Source: three-view drawing plus pictorial views. Frame: mm from the lowest corner of the part. Give positions to 0.01 mm unless a question says otherwise; leave off trailing zeros. Loops run counter-clockwise (first coordinate to the right, second up) from the corner with the lowest first, then second, coordinate; pieces in that order, holes last. Notation, with made-up numbers: (49.5, -28) - (92.5, -28) arc R19 ccw to (92.5, -5) - close; hole circle Ø8 at (9, 82). An arc over 180 degrees is marked (long way). Put each result on its own line as item: value.
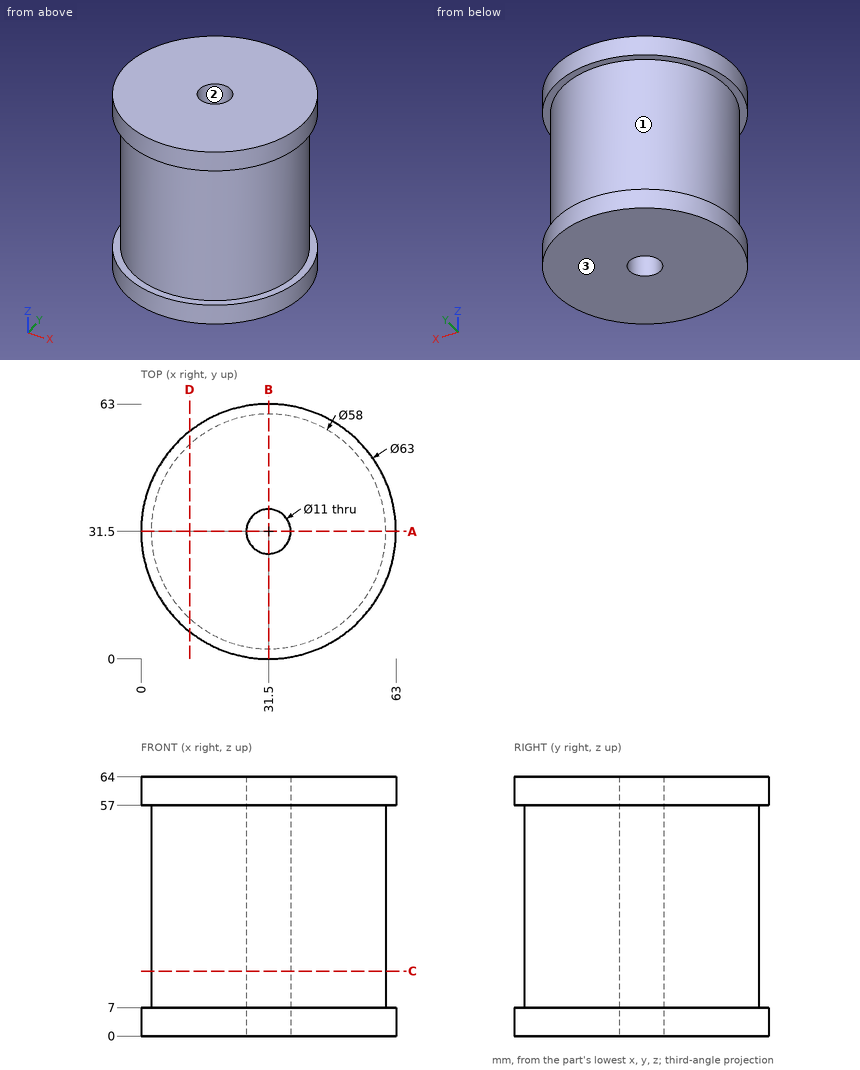
1) Pin query (flat end, axial travel): P1, Ø10, axis at x = 17.5, z = 10, coming from the -Y side; P2, Ø2, axis at y = 7.5, z = 27.5, coming from the +X side; P3, Ø1, axis at y = 25.5, z = 22, coming from the +X side; P4, Ø6.5, axis at x = 31.5, y = 31.5, coming from the -Z side. Return the tip coordinate at first contact, or that it passes through.
Check result:
P1: y = 1.63
P2: x = 49.16
P3: x = 59.97
P4: through
2) Section query A-A, the plane y = 31.5. Output: boundary loops of the cut face in (x, z).
Check result:
outline: (0, 0) - (26, 0) - (26, 64) - (0, 64) - (0, 57) - (2.5, 57) - (2.5, 7) - (0, 7) - close; (37, 0) - (63, 0) - (63, 7) - (60.5, 7) - (60.5, 57) - (63, 57) - (63, 64) - (37, 64) - close
3) Section query D-D, the plane x = 12. Output: boundary loops of the cut face in (y, z), plus the area to 3 significant figures.
Check result:
outline: (6.76, 0) - (56.24, 0) - (56.24, 7) - (52.97, 7) - (52.97, 57) - (56.24, 57) - (56.24, 64) - (6.76, 64) - (6.76, 57) - (10.03, 57) - (10.03, 7) - (6.76, 7) - close
area: 2,840 mm²
4) Section query C-C, the plane z = 16. Output: boundary loops of the cut face in (x, y).
Check result:
outline: circle Ø58 at (31.5, 31.5); hole circle Ø11 at (31.5, 31.5)
5) Material intervals for line 1 along Y through (x, z) = (31.5, 27.5); line 2 along Z through (x, y) = (56.5, 47); line 3 along X through (y, z) = (31, 24), sorted ascending. Write a range as [from, to].
Check result:
line 1: [2.5, 26], [37, 60.5]
line 2: [0, 7], [57, 64]
line 3: [2.5, 26.02], [36.98, 60.5]
6) Mould query, pull axis X, two halves, no side actions, for the marked faces 1, 2 and 3. Classes: pulls with the +X half, pulls with the -X half, needs draft (parallel to the pull), parting line crosses it, or undercut.
Check result:
face 1: parting line crosses it
face 2: undercut
face 3: needs draft
